Autodesk Inventor part; units mm, degrees
ref_plane "YZ Plane" through (0, 0, 0) normal (1, 0, 0) x (0, 1, 0)
ref_plane "XZ Plane" through (0, 0, 0) normal (0, 1, 0) x (-1, 0, 0)
ref_plane "XY Plane" through (0, 0, 0) normal (0, 0, 1) x (1, 0, 0)
sketch "スケッチ1" plane through (0, 0, 0) normal (0, 0, 1) x (1, 0, 0)
  circle A0 centre (0, 0) radius 40.5
  circle A1 centre (0, 440) radius 40.5
  line L0 (-40.5, 0) -> (-40.5, 440)
  line L1 (40.5, 440) -> (40.5, 0)
  dimension "d0" = 81
  dimension "d1" = 81
  dimension "d2" = 440
extrude "プレート1" add sketch "スケッチ1" along normal blind 2
sketch "スケッチ6" plane through (0, 0, 2) normal (0, 0, 1) x (1, 0, 0)
  arc A0 (40.5, 440) -> (-40.5, 440) centre (0, 440) ccw
  circle A1 centre (0, 440) radius 32.55
  point P0 (0, 0)
  dimension "d43" = 65.1
extrude "押し出し2" cut sketch "スケッチ6" against normal blind 10
sketch "スケッチ7" plane through (0, 0, 2) normal (0, 0, 1) x (1, 0, 0)
  arc A0 (40.5, 440) -> (-40.5, 440) centre (0, 440) ccw
  circle A1 centre (0, 440) radius 36.5
  point P0 (0, 0)
  point P1 (0, 476.5)
  point P2 (-31.6099, 458.25)
  point P3 (-31.6099, 421.75)
  point P4 (0, 403.5)
  point P5 (31.6099, 421.75)
  point P6 (31.6099, 458.25)
  dimension "d46" = 73
  dimension "d49" = 360
hole "穴4" at (0, 476.5, 2) at (-31.6099, 458.25, 2) at (-31.6099, 421.75, 2) at (0, 403.5, 2) at (31.6099, 421.75, 2) at (31.6099, 458.25, 2) direction (0, 0, -1) diameter 3.2 end through all
sketch "スケッチ8" plane through (0, 0, 2) normal (0, 0, 1) x (1, 0, 0)
  arc A0 (40.5, 440) -> (-40.5, 440) centre (0, 440) ccw
  circle A1 centre (0, 440) radius 25
  line L0 (23.4923, 431.4495) -> (-32.7335, 276.9703)
  line L1 (-23.4923, 448.5505) -> (-36.9957, 411.4503)
  line L2 (0, 603.9) -> (0, -147.9)
  circle A2 centre (0, 355.2097) radius 4
  point P0 (0, 0)
  point P1 (4, 72)
  dimension "d92" = 50
  dimension "d93" = 20
  dimension "d94" = 8
  dimension "d102" = 0
  dimension "d140" = 72
  dimension "d141" = 4
hole "穴5" at (4, 72, 2) at (0, 355.2097, 2) direction (0, 0, -1) diameter 4.3 end through all
sketch "スケッチ9" plane through (0, 0, 2) normal (0, 0, 1) x (1, 0, 0)
  circle A0 centre (0, 0) radius 67.5
  circle A1 centre (9, 84) radius 8
  arc A2 (40.5, 440) -> (-40.5, 440) centre (0, 440) ccw
  dimension "d69" = 84
  dimension "d79" = 135
  dimension "d80" = 16
  dimension "d144" = 9
hole "穴6" at (9, 84, 2) direction (0, 0, -1) diameter 4.3 end through all
sketch "スケッチ13" plane through (0, 0, 2) normal (0, 0, 1) x (1, 0, 0)
  circle A0 centre (0, 0) radius 15
  point P0 (0, 15)
  point P1 (-12.9904, 7.5)
  point P2 (-12.9904, -7.5)
  point P3 (0, -15)
  point P4 (12.9904, -7.5)
  point P5 (12.9904, 7.5)
  dimension "d109" = 30
  dimension "d112" = 360
hole "穴8" at (0, 15, 2) at (-12.9904, 7.5, 2) at (-12.9904, -7.5, 2) at (0, -15, 2) at (12.9904, -7.5, 2) at (12.9904, 7.5, 2) direction (0, 0, -1) diameter 3.2 end through all
sketch "スケッチ14" plane through (0, 0, 2) normal (0, 0, 1) x (1, 0, 0)
  circle A0 centre (0, 0) radius 10
  dimension "d121" = 20
extrude "押し出し5" cut sketch "スケッチ14" against normal blind 10
sketch "スケッチ15" plane through (0, 0, 2) normal (0, 0, 1) x (1, 0, 0)
  line L0 (-16, 84) -> (9, 84) construction
  line L1 (-16, 81.85) -> (9, 81.85)
  line L2 (9, 86.15) -> (-16, 86.15)
  arc A0 (-16, 86.15) -> (-16, 81.85) centre (-16, 84) ccw
  arc A1 (9, 81.85) -> (9, 86.15) centre (9, 84) ccw
  circle A2 centre (9, 84) radius 2.15
  point P0 (0, 0)
  dimension "d142" = 25
extrude "押し出し6" cut sketch "スケッチ15" against normal blind 10
sketch "スケッチ17" plane through (0, 0, 0) normal (0, 0, -1) x (-1, 0, 0)
  point P0 (0, 0)
  point P1 (0, 220)
  dimension "d132" = 220
hole "穴9" at (0, 220, 0) direction (0, 0, 1) diameter 4.3 end through all
sketch "スケッチ16" plane through (0, 0, 2) normal (0, 0, 1) x (1, 0, 0)
  line L0 (-21, 72) -> (4, 72) construction
  line L1 (-21, 69.85) -> (4, 69.85)
  line L2 (4, 74.15) -> (-21, 74.15)
  arc A0 (-21, 74.15) -> (-21, 69.85) centre (-21, 72) ccw
  arc A1 (4, 69.85) -> (4, 74.15) centre (4, 72) ccw
  circle A2 centre (4, 72) radius 2.15
  point P0 (0, 0)
  point P1 (-8.5, 72)
  dimension "d143" = 21
extrude "押し出し7" cut sketch "スケッチ16" against normal blind 10
equation "\"d56\" = Thickness"
equation "\"d67\" = Thickness"
equation "\"d77\" = Thickness"
equation "\"d119\" = Thickness"
equation "\"d138\" = Thickness"
equation "\"d3\" = Thickness"
equation "\"BendRadius\" = Thickness"
equation "\"BendReliefWidth\" = Thickness"
equation "\"BendReliefDepth\" = 0.5 * Thickness"
equation "\"CornerReliefSize\" = 4 * Thickness"
equation "\"MinimumRemnant\" = 2 * Thickness"
equation "\"TransitionRadius\" = BendRadius"
equation "\"JacobiRadiusSize\" = Thickness"
equation "\"GapSize\" = Thickness"
properties part number "link2-plate1" material "CFRP"
Source: CAD feature listing. Evaluate the final solid. Frame: model axes, mm. Round coordinates to 2 decimals unless told otherwise and drop trailing zeros. Write each loop counter-clockwise with the first axis right and the second up, starting at its lowest first coordinate (ties: lowest second). Pieces come first, ordered by that corner, then holes. Notation, with made-up numbers: M -14.75,44 L -4.75,44 A18 ccw -4.75,48 Z; hole C -17,16.5 d3. An arc over 180 degrees is marked long. Answer as a JSON object with one key per item and string values. Group by question number.
(1) Section query B-B on z = 0.85. State how many separate pieces and enclosed holes the cut face has, then the cut area to 3 significant figures.
(2) First-contact query: pin 1 (1 mm diameter, centred on x = -20.5, z = 0.5, fed in from -Y). Flat tip, straight axial feed; report the tip coordinate or a pass-through.
(3) Mould query, pull axis X, two halves, no side actions, for faces 1 (the cylindrical face through (-7.056, 408.224, 1.014)), 2 (the cylindrical face through (0.89, -40.49, 0.99)), 3 (the cylindrical face through (-2.17, -9.76, 1.01)), 4 (the flat face through (-1, 224, 2)). Classes: +X half, -X half, draft (parallel to the pull), parting line (faces both ways), or undercut.
(4) Ray query, line 1 (X direction, y = 421.75, z = 1.1); line 2 (X direction, y = 412, z = 0.55); line 3 (Y direction, x = 13, z = 1.2). Return the intervals inside material, ascending. Write a range as [from, to].
(5) Section query A-A on x = 21. Output: boundary loops of the cut face in (y, z), then the cut area to 3 significant figures.
Computed values:
{
 "1": {"separate pieces": "1", "enclosed holes": "18", "area": "36,800 mm^2"},
 "2": {"pin 1": "y = -35.22"},
 "3": {"face 1": "undercut", "face 2": "parting line", "face 3": "undercut", "face 4": "draft"},
 "4": {"line 1": "[-40.5, -33.21], [-30.01, -26.95], [26.95, 30.01], [33.21, 40.5]", "line 2": "[-40.5, -16.6], [16.6, 40.5]", "line 3": "[-38.36, -9.1], [-5.9, 5.9], [9.1, 410.16], [469.84, 478.36]"},
 "5": {"outline": "M -34.63,0 L 415.13,0 L 415.13,2 L -34.63,2 Z; M 464.87,0 L 474.63,0 L 474.63,2 L 464.87,2 Z", "area": "919 mm^2"}
}
